Check sheet for the modelled part. Datum: model origin and axes. Units: mm. Round coordinates to 2 decimals unless told otherwise and drop trailing zeros. Write each loop counter-clockwise with the first axis right and the second up, starting at its lowest first coordinate (ties: lowest second). Pieces come first, ordered by that corner, then holes.
Item 1: Go/stop test with flat-tipped pins: pin 1 Ø2 at (x, z) = (3.5, 1.5) entering from +Y; pin 2 Ø1.5 at (y, z) = (42.5, 4.5) entering from -X. Record where each tip stops, or that it passes through.
Item 2: Cross-section at B-B on y = 22. Enter the section's corners in (x, z), plus the area to 3 significant figures.
Item 3: Cross-section at A-A on x = 0. Enter the section's corners in (y, z), plus the area to 3 significant figures.
Item 4: Material ranges on line 1 (X direction, y = -10.5, z = 1.75); line 2 (Y direction, x = 0, z = 1.5); line 3 (Y direction, x = 69.5, z = 6), recorded low to high.
Item 5: Release check for a two-part mould opening along X. For faces 1 (the cylindrical face through (0.715, 63.496, 3.131)), 2 (the cylindrical face through (-64.3, 3.81, 3.13)), 3 (the flat face through (46, 1, 0)) record: +X half, -X half, draft (parallel to the pull), parting line (faces both ways), or undercut.
Item 6: Cross-section at C-C on y = 9. Enter the section's corners in (x, z).
Item 7: Cross-section at D-D on z = 1. Count the separate pieces of the cut face and the enclosed holes in it, plus the area to 3 significant figures.
from build123d import *

# Parameters (mm, degrees)
F0_R     = 12.7
F1_DEPTH = 6.35
F2_R     = 38.1


# Not quite as in the source:
# - a length typed as a fraction of an inch, garbled in the dataset ("3 / 203.2 mm" for 3/8 in), is restored


with BuildPart() as f1:
    # F0 (on Top) → F1 (new body)
    with BuildSketch(Plane.XY):
        with BuildLine():
            ThreePointArc((44.2896283804, 3.7724419046), (44.4098889973, 1.8879245867), (44.45, 0))
            ThreePointArc((44.45, 0), (44.4098889973, -1.8879245867), (44.2896283804, -3.7724419046))
            ThreePointArc((44.2896283804, -3.7724419046), (48.6524538165, -16.4400117074), (57.8519523886, -26.1801757984))
            ThreePointArc((57.8519523886, -26.1801757983), (61.7568132692, -14.7765359551), (63.4364387448, -2.8404646402))
            ThreePointArc((63.4364387448, -2.8404646402), (63.1147165179, 0), (63.4364387448, 2.8404646402))
            ThreePointArc((63.4364387448, 2.8404646402), (61.7568132692, 14.7765359551), (57.8519523886, 26.1801757983))
            ThreePointArc((57.8519523886, 26.1801757984), (48.6524538165, 16.4400117074), (44.2896283804, 3.7724419046))
        make_face()
        with BuildLine():
            ThreePointArc((44.2896283804, -3.7724419046), (-44.45, 0), (44.2896283804, 3.7724419046))
            ThreePointArc((44.2896283804, 3.7724419046), (48.6524538165, 16.4400117074), (57.8519523886, 26.1801757984))
            ThreePointArc((57.8519523886, 26.1801757983), (-0.1747733497, 63.499759482), (-57.9951886366, 25.8613243088))
            ThreePointArc((-57.9951886366, 25.8613243088), (-48.1929456979, 14.5475718573), (-44.6640486717, 0))
            ThreePointArc((-44.6640486717, 0), (-48.1929456979, -14.5475718573), (-57.9951886366, -25.8613243088))
            ThreePointArc((-57.9951886366, -25.8613243088), (-0.1747733497, -63.499759482), (57.8519523886, -26.1801757983))
            ThreePointArc((57.8519523886, -26.1801757984), (48.6524538165, -16.4400117074), (44.2896283804, -3.7724419046))
        make_face()
        with BuildLine():
            ThreePointArc((107.5647165179, 0), (90.6090522396, 28.09252802), (57.8519523886, 26.1801757984))
            ThreePointArc((57.8519523886, 26.1801757983), (61.7568132692, 14.7765359551), (63.4364387448, 2.8404646402))
            ThreePointArc((63.4364387448, 2.8404646402), (77.244029689, 12.6193131294), (88.5147165179, 0))
            ThreePointArc((88.5147165179, 0), (77.244029689, -12.6193131294), (63.4364387448, -2.8404646402))
            ThreePointArc((63.4364387448, -2.8404646402), (61.7568132692, -14.7765359551), (57.8519523886, -26.1801757983))
            ThreePointArc((57.8519523886, -26.1801757984), (90.6090522396, -28.09252802), (107.5647165179, 0))
        make_face()
        with BuildLine():
            ThreePointArc((-44.6640486717, 0), (-48.1929456979, 14.5475718573), (-57.9951886366, 25.8613243088))
            ThreePointArc((-57.9951886366, 25.8613243088), (-63.5, 0), (-57.9951886366, -25.8613243088))
            ThreePointArc((-57.9951886366, -25.8613243088), (-48.1929456979, -14.5475718573), (-44.6640486717, 0))
        make_face()
        with BuildLine():
            ThreePointArc((-57.9951886366, -25.8613243088), (-63.5, 0), (-57.9951886366, 25.8613243088))
            ThreePointArc((-57.9951886366, 25.8613243088), (-108.1640486717, 0), (-57.9951886366, -25.8613243088))
        make_face()
        with Locations((-76.4140486717, 0)):
            Circle(F0_R, mode=Mode.SUBTRACT)
    extrude(amount=F1_DEPTH)

    # F2
    f2_edges = [f1.edges().sort_by_distance(p)[0] for p in [
        (-57.995189, 25.861324, 3.175),
        (57.851952, 26.180176, 3.175),
        (-57.995189, -25.861324, 3.175),
        (57.851952, -26.180176, 3.175),
    ]]
    fillet(f2_edges, radius=F2_R)


solid = f1.part
Response values:
1. pin 1: stops at y = 63.45
1. pin 2: stops at x = -48.04
2. outline: (-99.31, 0) - (-38.62, 0) - (-38.62, 6.35) - (-99.31, 6.35) - close; (38.62, 0) - (98.71, 0) - (98.71, 6.35) - (38.62, 6.35) - close
2. area: 767 mm2
3. outline: (-63.5, 0) - (-44.45, 0) - (-44.45, 6.35) - (-63.5, 6.35) - close; (44.45, 0) - (63.5, 0) - (63.5, 6.35) - (44.45, 6.35) - close
3. area: 242 mm2
4. line 1: x = -106.38 to -83.56, -69.27 to -43.19, 43.19 to 68.67, 82.96 to 105.78
4. line 2: y = -63.5 to -44.45, 44.45 to 63.5
4. line 3: y = -31.97 to -11.02, 11.02 to 31.97
5. face 1: parting line
5. face 2: undercut
5. face 3: draft
6. outline: (-106.86, 0) - (-85.37, 0) - (-85.37, 6.35) - (-106.86, 6.35) - close; (-67.45, 0) - (-43.53, 0) - (-43.53, 6.35) - (-67.45, 6.35) - close; (43.53, 0) - (66.85, 0) - (66.85, 6.35) - (43.53, 6.35) - close; (84.78, 0) - (106.26, 0) - (106.26, 6.35) - (84.78, 6.35) - close
7. separate pieces: 1
7. enclosed holes: 3
7. area: 10,700 mm2
